For this review, take the finished solid that the model builds, in its own axes (mm). A direction names the side the tool comes from. Give positions to 0.01 mm unless a question says otherwise; leave off trailing zeros. Loops run counter-clockwise (first coordinate to the right, second up) from the corner with the lowest first, then second, coordinate; pieces in that order, holes last. Notation, with made-up numbers: (8, 6) -> (18, 6) arc R21 ccw to (18, 12) -> close; hole circle Ø8 at (53, -8.5). An arc over 180 degrees is marked (long way). Answer as CSV lines item,"result". Start each with the question number.
Item 1: Add section D-D on z = 45.5. State the section outline as (x, y) points (3 decimals).
Item 2: Add section B-B on x = 6.35. State the section outline as (y, z) points.
Item 3: Add section A-A on z = 11.43. State the section outline as (x, y) points.
Item 4: Clearance check with flat-ended pins moving along their axes: P1, Ø11, axis at y = -30.5, z = 65, coming from the -X side; P2, Ø4, axis at y = -23, z = 7.5, coming from the -X side; P3, Ø12, axis at x = 7.5, y = -30.5, coming from the -Z side; P4, Ø8, axis at x = 99, z = 50.5, coming from the +Y side. State where each tip first meets the part, or that it passes through.
Item 5: Machinability: for faces 1 (the face through (12, -22, 76.2)), 2 (the face through (11, -22, 13.97)), 3 (the face through (11, -22, 27.94)), which of the approach directions +Z, -Z, +X, -X, +Y, -Y give a long, thin tool a straight path to every point of the face, cutting with its end or side? Answer none if there is none.
Item 6: The part is to be moulded in two halves that separate along X. For faces 4 (the face through (80.743, -22.536, 12.861)), 5 (the face through (0.596, -19.252, 48.993)), 6 (the face through (9, -22, 69.85)), say which applies: +X half, -X half, draft (parallel to the pull), parting line (faces both ways), or undercut.
Item 7: For L1, parallel to Z at x = 15, y = -39.5; L2, parallel to Z at x = 141.5, y = -30.5; L3, parallel to X at y = -29.5, z = 58, list the stretches that pass through material, from the lowest coordinate up. Write a range as from..to.
```python
from build123d import *

# Parameters (mm, degrees)
F0_W       = 152.4
F0_H       = 76.2
F1_DEPTH   = 44.45
F2_W       = 15.24
F2_H       = 13.97
F3_DEPTH   = 44.451
F4_R       = 3.175
F5_DEPTH   = 69.85
F6_C1_SIZE = 19.05
F6_C2_SIZE = 19.05
F7_R       = 4.7625
F8_DEPTH   = 44.451
F10_DEPTH  = 44.45
F11_R      = 7.62


with BuildPart() as f1:
    # F0 (on Front) → F1 (new body)
    with BuildSketch(Plane.XZ):
        with Locations((76.2, 38.1)):
            Rectangle(F0_W, F0_H)
    extrude(amount=F1_DEPTH)

    # F2 (on face) → F3 (cut, through all)
    with BuildSketch(Plane.XZ.offset(44.45)):
        with Locations((7.62, 6.985)):
            Rectangle(F2_W, F2_H)
        with Locations((7.62, 34.925)):
            Rectangle(F2_W, F2_H)
        with Locations((7.62, 62.865)):
            Rectangle(F2_W, F2_H)
    extrude(amount=-F3_DEPTH, mode=Mode.SUBTRACT)

    # F4 (on face) → F5 (cut)
    with BuildSketch(Plane(origin=(0, 0, 0), x_dir=(1, 0, 0), z_dir=(0, 0, -1))):
        with Locations((6.35, 22.225)):
            Circle(F4_R)
    extrude(amount=-F5_DEPTH, mode=Mode.SUBTRACT)

    # F6: chamfer of 19.05 on 6 edges, made by hand

    # F6_c1
    f6_c1_edges = [f1.edges().sort_by_distance(p)[0] for p in [
        (0, 0, 73.025),
    ]]
    chamfer(f6_c1_edges, length=F6_C1_SIZE)

    # F6_c2
    f6_c2_edges = [f1.edges().sort_by_distance(p)[0] for p in [
        (0, -44.45, 73.025),
    ]]
    chamfer(f6_c2_edges, length=F6_C2_SIZE)

    # F7 (on face) → F8 (cut, through all)
    with BuildSketch(Plane.XZ.offset(44.45)):
        with Locations((76.2, 11.43)):
            Circle(F7_R)
    extrude(amount=-F8_DEPTH, mode=Mode.SUBTRACT)

    # F9 (on face) → F10 (join)
    with BuildSketch(Plane.XZ.offset(44.45)):
        Polygon((23.4944241071, 127), (19.05, 76.2), (76.2, 76.2), (76.2, 127), align=None)
    extrude(amount=-F10_DEPTH)

    # F11
    f11_edges = [f1.edges().sort_by_distance(p)[0] for p in [
        (0, -19.05, 73.025),
        (0, -25.4, 73.025),
        (0, -25.4, 48.895),
        (0, -19.05, 48.895),
        (0, -19.05, 20.955),
        (0, -25.4, 20.955),
    ]]
    fillet(f11_edges, radius=F11_R)


solid = f1.part
```
Computed values:
1,outline,"(0, -22.244) arc R7.62 ccw to (2.232, -27.632) -> (19.05, -44.45) -> (152.4, -44.45) -> (152.4, 0) -> (19.05, 0) -> (2.232, -16.818) arc R7.62 ccw to (0, -22.206) -> close; hole circle Ø6.35 at (6.35, -22.225)"
2,outline,"(-31.75, 13.97) -> (-25.4, 13.97) -> (-25.4, 27.94) -> (-31.75, 27.94) -> close; (-31.75, 41.91) -> (-25.4, 41.91) -> (-25.4, 55.88) -> (-31.75, 55.88) -> close; (-31.75, 69.85) -> (-12.7, 69.85) -> (-12.7, 76.2) -> (-31.75, 76.2) -> close; (-19.05, 13.97) -> (-12.7, 13.97) -> (-12.7, 27.94) -> (-19.05, 27.94) -> close; (-19.05, 41.91) -> (-12.7, 41.91) -> (-12.7, 55.88) -> (-19.05, 55.88) -> close"
3,outline,"(15.24, -40.64) -> (19.05, -44.45) -> (71.44, -44.45) -> (71.44, 0) -> (19.05, 0) -> (15.24, -3.81) -> close; (80.96, -44.45) -> (152.4, -44.45) -> (152.4, 0) -> (80.96, 0) -> close"
4,P1,"x = 2.51"
4,P2,"x = 15.24"
4,P3,"z = 13.97"
4,P4,"y = 0"
5,face 1,"+Z, -X, +Y, -Y"
5,face 2,"-Z, -X, +Y, -Y"
5,face 3,"-X, +Y, -Y"
6,face 4,"undercut"
6,face 5,"-X half"
6,face 6,"draft"
7,L1,"13.97..27.94, 41.91..55.88, 69.85..76.2"
7,L2,"0..76.2"
7,L3,"15.24..152.4"
